For this review, take the finished solid that the model builds, in its own axes (mm). A direction names the side the tool comes from. Give positions to 0.01 mm unless a question says otherwise; leave off trailing zeros. Order: outer loops, then holes, each group sorted by start corner. A loop starts at its lowest first (then second) coordinate and runs counter-clockwise, first axis right, second up.
Item 1: Consider section B-B (z = -5). Give the boundary of the cut face in (x, y).
Item 2: Consider section C-C (x = 1.9). Give the number of separate pieces and of enclosed holes in the cut face, plus the area to 3 significant figures.
Item 3: The part is to be moulded in two halves that separate along Z. For faces 3 (the flat face through (1, 29.412, -2)), 4 (the cylindrical face through (1.479, -26.146, 4.721)), 5 (the cylindrical face through (1.479, 24.916, 11.324)), say which applies: released by +Z, released by -Z, zero draft, split by the parting line, or undercut.
Item 4: For probe 1 along Y at (x, z) = (2.05, -5); probe 2 along Y at (x, z) = (2.25, 4.5); probe 3 along Z at (x, y) = (2.55, -24.5), list the stretches that pass through material, from the lowest coordinate up.
Item 5: Machinability: for faces 1 (the cylindrical face through (1.479, 25.942, -4.075)), 2 (the flat face through (1, 0, -11.525)), which of the approach directions +Z, -Z, +X, -X, +Y, -Y give a long, thin tool a straight path to every point of the face, cutting with its end or side? Answer none if there is none.
Item 6: Consider section A-A (y = 0). Give the boundary of the cut face in (x, z) (3 decimals).
Item 7: For P1, Ø2.5, axis at y = -126.56, z = -27.41, coming from the +X side; P2, Ø4.5, axis at y = -24.21, z = 4.97, coming from the +X side; P3, Ø1, axis at x = 1, y = -66, coming from the +Z side, all flat-tipped, find the tip position at first contact; note any pin that passes through.
Item 8: Consider section D-D (y = -18). Give the boundary of the cut face in (x, z) (3 decimals).
```python
from build123d import *

# Parameters (mm, degrees)
SKETCH1_R           = 1.95
SKETCH1_R_2         = 1.5
BOSS_EXTRUDE1_DEPTH = 3


with BuildPart() as part:
    # Sketch1 → Boss-Extrude1 (new body)
    with BuildSketch(Plane(origin=(0, 0, 0), x_dir=(0, 0, -1), z_dir=(1, 0, 0))):
        with BuildLine():
            Line((-6.925, 29.4125), (11.525, 29.4125))
            ThreePointArc((11.525, 29.4125), (16.101209281, 28.129035679), (19.342554621, 24.653024687))
            ThreePointArc((19.342554621, 24.653024687), (40.969128184, -50.437912981), (32.171039161, -128.084234422))
            ThreePointArc((32.171039161, -128.084234422), (25.983785002, -131.35426762), (22.587628574, -125.235333672))
            ThreePointArc((22.587628574, -125.235333672), (27.867812209, -90.719506549), (25.024864397, -55.91806536))
            ThreePointArc((25.024864397, -55.91806536), (13.295850828, -37.309652467), (-7.219256672, -29.374089856))
            ThreePointArc((-7.219256672, -29.374089856), (-11.325, -24.983940313), (-7.219256672, -20.59379077))
            Line((-7.219256672, -20.59379077), (11.525, -20.59379077))
            Line((11.525, -20.59379077), (11.525, 20.6125))
            Line((11.525, 20.6125), (-6.925, 20.6125))
            ThreePointArc((-6.925, 20.6125), (-11.325, 25.0125), (-6.925, 29.4125))
        make_face()
        with Locations((-4.975, 24.2125)):
            Circle(SKETCH1_R, mode=Mode.SUBTRACT)
        with Locations(Location((4.975, 24.2125, 0), (0, 0, 180))):
            Circle(SKETCH1_R, mode=Mode.SUBTRACT)
        with Locations((4.975, -24.2125)):
            Circle(SKETCH1_R, mode=Mode.SUBTRACT)
        with Locations(Location((-4.975, -24.2125, 0), (0, 0, 180))):
            Circle(SKETCH1_R, mode=Mode.SUBTRACT)
        with Locations((18.795, 0)):
            Circle(SKETCH1_R_2, mode=Mode.SUBTRACT)
        with Locations((33.159858862, -55.41852876)):
            Circle(SKETCH1_R_2, mode=Mode.SUBTRACT)
        with Locations((32.663736784, -107.316157442)):
            Circle(SKETCH1_R_2, mode=Mode.SUBTRACT)
        with Locations((30.036135717, -116.938856525)):
            Circle(SKETCH1_R_2, mode=Mode.SUBTRACT)
        with Locations((27.408534649, -126.561555607)):
            Circle(SKETCH1_R_2, mode=Mode.SUBTRACT)
    extrude(amount=BOSS_EXTRUDE1_DEPTH)


solid = part.part
```
Resolved:
1. outline: (0, -32.23) - (3, -32.23) - (3, -26.16) - (0, -26.16) - close; (0, -22.26) - (3, -22.26) - (3, -20.59) - (0, -20.59) - close; (0, 20.61) - (3, 20.61) - (3, 22.26) - (0, 22.26) - close; (0, 26.16) - (3, 26.16) - (3, 29.41) - (0, 29.41) - close
2. separate pieces: 1
2. enclosed holes: 9
2. area: 2,900 mm2
3. face 3: zero draft
3. face 4: undercut
3. face 5: released by +Z
4. probe 1: y = -32.23 to -26.16, -22.26 to -20.59, 20.61 to 22.26, 26.16 to 29.41
4. probe 2: y = -29.62 to -26.1, -22.32 to -20.59, 20.61 to 22.32, 26.1 to 29.41
4. probe 3: z = -37.06 to -6.9, -3.05 to 3.05, 6.9 to 11.3
5. face 1: +X, -X
5. face 2: +Z, +X, -X
6. outline: (0, -30.051) - (3, -30.051) - (3, -20.295) - (0, -20.295) - close; (0, -17.295) - (3, -17.295) - (3, -11.525) - (0, -11.525) - close
7. P1: passes through
7. P2: stops at x = 3
7. P3: stops at z = -26.63
8. outline: (0, -35.531) - (3, -35.531) - (3, -11.525) - (0, -11.525) - close
